```python
from build123d import *

# Parameters (mm, degrees)
BOSS_EXTRUDE1_DEPTH = 15
SKETCH2_W           = 7.335
SKETCH2_H           = 6
CUT_EXTRUDE1_DEPTH  = 14
SKETCH2_3_R         = 1.5
CUT_EXTRUDE2_DEPTH  = 27.937700811


with BuildPart() as part:
    # Sketch1 → Boss-Extrude1 (new body)
    with BuildSketch(Plane.XY):
        with BuildLine():
            Line((0, -2), (-14.835, -2))
            Line((-14.835, -2), (-14.835, 7.415))
            ThreePointArc((-14.835, 7.415), (-12.68662824, 12.60162824), (-7.5, 14.75))
            Line((-7.5, 14.75), (7.5, 14.75))
            ThreePointArc((7.5, 14.75), (12.68662824, 12.60162824), (14.835, 7.415))
            Line((14.835, 7.415), (14.835, -2))
            Line((14.835, -2), (0, -2))
        make_face()
        with BuildLine():
            Line((-5, 6.75), (-5, 5))
            ThreePointArc((-5, 5), (0, 0), (5, 5))
            Line((5, 5), (5, 6.75))
            ThreePointArc((5, 6.75), (0, 11.75), (-5, 6.75))
        make_face(mode=Mode.SUBTRACT)
    extrude(amount=-BOSS_EXTRUDE1_DEPTH)

    # Sketch2 → Cut-Extrude1 (cut)
    with BuildSketch(Plane(origin=(0, 14.75, 0), x_dir=(1, 0, 0), z_dir=(0, 1, 0))):
        with Locations((-11.1675, 7.5)):
            Rectangle(SKETCH2_W, SKETCH2_H)
    cut_extrude1 = extrude(amount=-CUT_EXTRUDE1_DEPTH, mode=Mode.SUBTRACT)

    # Sketch2_3 → Cut-Extrude2 (cut, through all)
    with BuildSketch(Plane(origin=(0, 14.75, 0), x_dir=(1, 0, 0), z_dir=(0, 1, 0))):
        with Locations(Location((-10.54250606, 7.5, 0), (0, 0, 270))):
            Circle(SKETCH2_3_R)
    cut_extrude2 = extrude(amount=-CUT_EXTRUDE2_DEPTH, mode=Mode.SUBTRACT)

    # Mirror1: Cut-Extrude1, Cut-Extrude2 across plane
    add(cut_extrude1.mirror(Plane(origin=(0, 0, 0), x_dir=(0, 0, 1), z_dir=(1, 0, 0))), mode=Mode.SUBTRACT)
    add(cut_extrude2.mirror(Plane(origin=(0, 0, 0), x_dir=(0, 0, 1), z_dir=(1, 0, 0))), mode=Mode.SUBTRACT)


solid = part.part
```
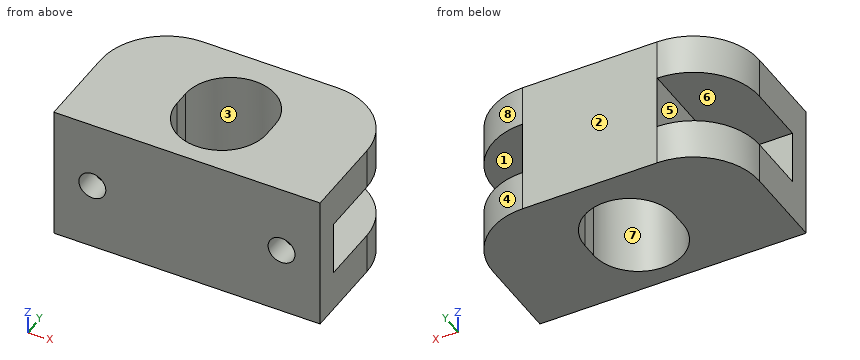
The model under review builds one solid part; all positions refer to its coordinate system, in mm. Face numbers are marked on the shaded views. A direction names the side the tool comes from. Give positions to 0.01 mm unless a question says otherwise; leave off trailing zeros. Write each loop counter-clockwise with the first axis right and the second up, starting at its lowest first coordinate (ties: lowest second). Pieces come first, ordered by that corner, then holes. Notation, with made-up numbers: (73.25, -24) -> (118.25, -24) arc R13 ccw to (118.25, -6) -> close; hole circle Ø4 at (-16, -21.75). An arc over 180 degrees is marked (long way). Put each result on its own line as item: value.
(1) We need section B-B, the plane x = 4. Give the boundary of the cut face in (y, z).
Results are:
outline: (-2, -15) -> (2, -15) -> (2, 0) -> (-2, 0) -> close; (9.75, -15) -> (14.75, -15) -> (14.75, 0) -> (9.75, 0) -> close
(2) We need section A-A, the plane z = -7.5. State how many separate pieces and enclosed holes the cut face has, and give its area (3 significant figures).
Results are:
separate pieces: 3
enclosed holes: 1
area: 179 mm²
(3) We need section D-D, the plane y = 1.5. Give the boundary of the cut face in (x, z) (3 decimals), and give its area (3 significant figures).
Results are:
outline: (-14.835, -15) -> (-3.571, -15) -> (-3.571, 0) -> (-14.835, 0) -> (-14.835, -4.5) -> (-7.5, -4.5) -> (-7.5, -10.5) -> (-14.835, -10.5) -> close; (3.571, -15) -> (14.835, -15) -> (14.835, -10.5) -> (7.5, -10.5) -> (7.5, -4.5) -> (14.835, -4.5) -> (14.835, 0) -> (3.571, 0) -> close
area: 250 mm²
(4) For pin 1 Ø1.9 at (y, z) = (6.5, -6.5) entering from +X; pin 2 Ø3.5 at (x, z) = (10.54, -7.5) entering from +Y; pin 3 Ø4 at (y, z) = (13, -12.5) entering from +X, all flat-tipped, find the tip position at first contact; note any pin that passes through.
Results are:
pin 1: x = 7.5
pin 2: y = 0.75
pin 3: x = 13.9
(5) We need section C-C, the plane z = -13. Give the boundary of the cut face in (x, y) (3 decimals).
Results are:
outline: (-14.835, -2) -> (14.835, -2) -> (14.835, 7.415) arc R7.335 ccw to (7.5, 14.75) -> (-7.5, 14.75) arc R7.335 ccw to (-14.835, 7.415) -> close; hole (-5, 5) arc R5 ccw to (5, 5) -> (5, 6.75) arc R5 ccw to (-5, 6.75) -> close
(6) To check wall thickness, follow probe 1 along X at (y, z) = (-0.65, -7.5) (1 decimal); probe 2 along Z at (x, y) = (-13.25, 3.75); probe 3 along X at (y, z) = (5.25, -2.25) (3 decimals). State the ranges of each line that lie inside material, in increasing order. Write a range as from..to.
Results are:
probe 1: -14.8..-12, -9..9, 12..14.8
probe 2: -15..-10.5, -4.5..0
probe 3: -14.835..-5, 5..14.835
(7) Tool access review of the marked faces 1, 2, 3, 4 and 5: name each direction out of +Z, -Z, +X, -X, +Y, -Y from which nothing blocks a thin tool from reaching the whole face with its end or side.
Results are:
face 1: +X, +Y
face 2: +Z, -Z, +X, -X, +Y
face 3: +Z, -Z
face 4: +Z, -Z, +X, +Y
face 5: -X, +Y
(8) The part is to be moulded in two halves that separate along X. For the marked faces 6, 7 and 8, say which applies: pulls with the +X half, pulls with the -X half, needs draft (parallel to the pull), parting line crosses it, or undercut.
Results are:
face 6: needs draft
face 7: undercut
face 8: pulls with the +X half
